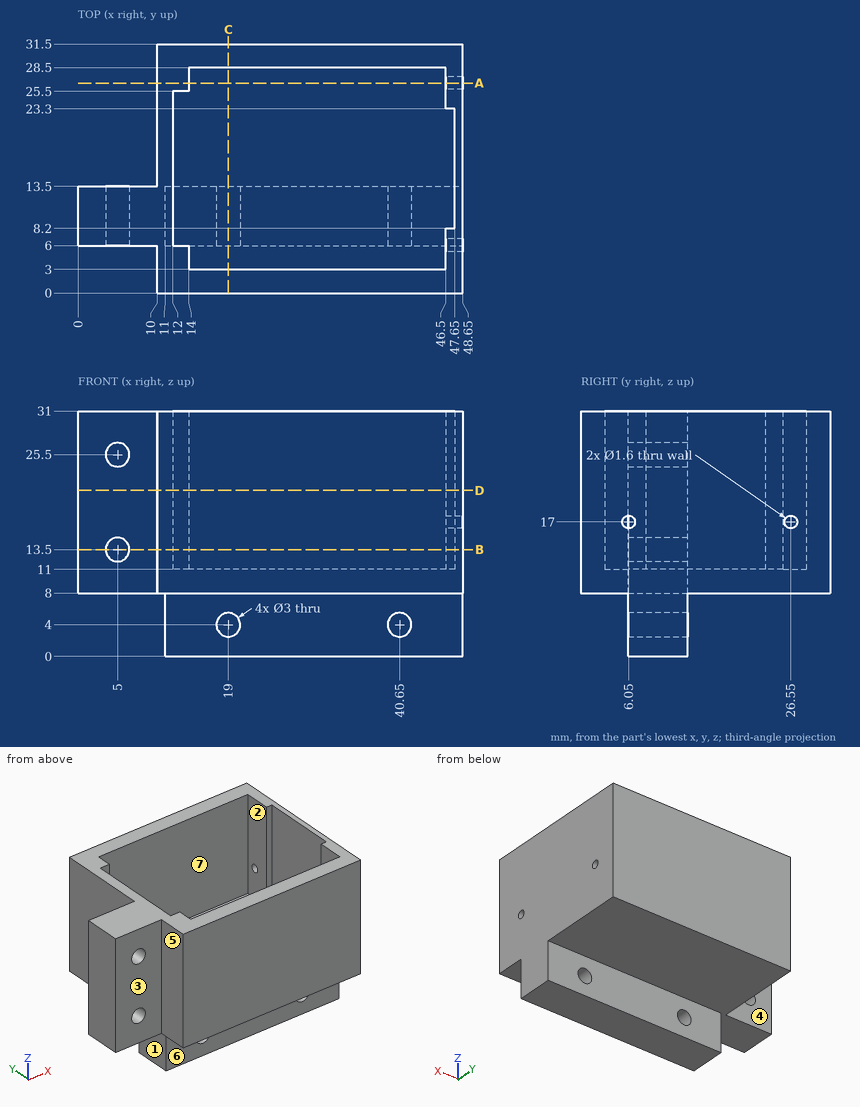
Check sheet for the drawn part. Datum: minimum x, y, z corner. Units: mm. A direction names the side the tool comes from. Round coordinates to 2 decimals unless told otherwise and drop trailing zeros. Loops run counter-clockwise (first coordinate to the right, second up) from the corner with the lowest first, then second, coordinate; pieces in that order, holes last. Notation, with made-up numbers: M 8.5,-15.5 L 43.5,-15.5 A22 cw 43.5,3.5 Z; hole C 47.5,25 d8. An arc over 180 degrees is marked long. Write each question's results on one line, items separated by ' | '.
1) Scan lines: L1, parallel to X at y = 9, z = 4; L2, parallel to X at y = 10.25, z = 25.5; L3, parallel to Y at x = 18, z = 16. Record each from-to range of solid material in increasing order. Write a range as from..to.
Checks:
L1: x = 11..17.5, 20.5..39.15, 42.15..48.65 | L2: x = 0..3.5, 6.5..12, 47.65..48.65 | L3: y = 0..3, 28.5..31.5
2) Mould release check, pull along X, two halves, no side actions. Record for the marked faces 5, 6 and 7: released by +X, released by -X, zero draft, split by the parting line, or undercut.
Checks:
face 5: released by -X | face 6: zero draft | face 7: undercut
3) Access from +Z, -Z, +X, -X, +Y, -Y to the whole of each face (thin tool, end or side, straight path). Record for the marked faces 1, 2, 3 and 4.
Checks:
face 1: -Z, -X, +Y, -Y | face 2: +Z | face 3: +Z, -Z, -X, -Y | face 4: +Z, -Z, -X, +Y
4) Section check C-C on x = 19. Record the boundary of the cut face in (y, z).
Checks:
outline: M 0,8 L 6,8 L 6,5.5 L 13.5,5.5 L 13.5,8 L 31.5,8 L 31.5,31 L 28.5,31 L 28.5,11 L 3,11 L 3,31 L 0,31 Z; M 6,0 L 13.5,0 L 13.5,2.5 L 6,2.5 Z
5) Section check D-D on z = 21. Record the boundary of the cut face in (x, y), then the cut area to 3 significant figures.
Checks:
outline: M 0,6 L 10,6 L 10,0 L 48.65,0 L 48.65,31.5 L 10,31.5 L 10,13.5 L 0,13.5 Z; hole M 12,6 L 14,6 L 14,3 L 46.5,3 L 46.5,8.2 L 47.65,8.2 L 47.65,23.3 L 46.5,23.3 L 46.5,28.5 L 14,28.5 L 14,25.5 L 12,25.5 Z | area: 407 mm2
6) Gauge pin test, flat ends, axial feed: P1, Ø1.4, axis at y = 26.55, z = 17, coming from the -X side; P2, Ø4, axis at x = 23.5, z = 3, coming from the +Y side; P3, Ø1.5, axis at y = 10, z = 4, coming from the -X side. Record the tip position at first contact, or that the pin passes through.
Checks:
P1: stops at x = 10 | P2: stops at y = 13.5 | P3: stops at x = 11
7) Section check A-A on y = 26.55. Record the boundary of the cut face in (x, z).
Checks:
outline: M 10,8 L 48.65,8 L 48.65,16.2 L 46.5,16.2 L 46.5,11 L 14,11 L 14,31 L 10,31 Z; M 46.5,17.8 L 48.65,17.8 L 48.65,31 L 46.5,31 Z
8) Section check B-B on z = 13.5. Record the boundary of the cut face in (x, y), then the cut area to 3 significant figures.
Checks:
outline: M 0,6 L 3.5,6 L 3.5,13.5 L 0,13.5 Z; M 6.5,6 L 10,6 L 10,0 L 48.65,0 L 48.65,31.5 L 10,31.5 L 10,13.5 L 6.5,13.5 Z; hole M 12,6 L 14,6 L 14,3 L 46.5,3 L 46.5,8.2 L 47.65,8.2 L 47.65,23.3 L 46.5,23.3 L 46.5,28.5 L 14,28.5 L 14,25.5 L 12,25.5 Z | area: 385 mm2
